Here's how the part is built. I have some questions about the finished solid (model axes, mm). Round coordinates to 2 decimals unless told otherwise and drop trailing zeros. Order: outer loops, then holes, each group sorted by start corner. A loop starts at its lowest first (then second) coordinate and runs counter-clockwise, first axis right, second up. Notation, with made-up numbers: (43.5, 79.5) -> (61.5, 79.5) arc R30 cw to (61.5, 118.5) -> close; hole circle Ø3 at (38, 79). An arc over 180 degrees is marked (long way). Answer in a Markdown table with one row per item.
```python
from build123d import *

# Parameters (mm, degrees)
SKETCH1_R               = 5.5499
EXTRUDE1_DEPTH          = 4.7625
SKETCH7_OUTSIDE_W       = 113.114
SKETCH7_OUTSIDE_H       = 115.816
SKETCH7_OUTSIDE_R       = 8.73125
EXTRUDE2_DEPTH          = 25.4
EXTRUDE2_DRAFT          = -60
MIRROR1_COPY_1_SKETCH_W = 113.114
MIRROR1_COPY_1_SKETCH_H = 115.816
MIRROR1_COPY_1_SKETCH_R = 8.73125
MIRROR1_COPY_1_DEPTH    = 25.4
MIRROR1_COPY_1_DRAFT    = -60


with BuildPart() as part:
    # Sketch1 → Extrude1 (new, symmetric)
    with BuildSketch(Plane.XY):
        Polygon((-8.73125, 5.040989538), (-8.73125, -5.040989538), (0, -10.081979076), (8.73125, -5.040989538), (8.73125, 5.040989538), (0, 10.081979076), align=None)
        with Locations(Location((0, 0, 0), (0, 0, 180))):
            Circle(SKETCH1_R, mode=Mode.SUBTRACT)
    extrude(amount=EXTRUDE1_DEPTH, both=True)


with BuildPart() as extrude2_tool:
    # Sketch7 outside → Extrude2 (with draft: the straight prism first)
    with BuildSketch(Plane.XY.offset(4.7625)):
        Rectangle(SKETCH7_OUTSIDE_W, SKETCH7_OUTSIDE_H)
        Circle(SKETCH7_OUTSIDE_R, mode=Mode.SUBTRACT)
    extrude(amount=-EXTRUDE2_DEPTH)
    # Extrude2: the draft: its side faces are tilted about the plane it starts from
    extrude2_sides = [extrude2_tool.faces().sort_by_distance(p)[0] for p in [
        (0, -57.908, -7.9375),
        (56.557, 0, -7.9375),
        (0, 57.908, -7.9375),
        (-56.557, 0, -7.9375),
        (-8.73125, 0, -7.9375),
    ]]
    draft(extrude2_sides, Plane.XY.offset(4.7625), EXTRUDE2_DRAFT)


with BuildPart() as part_1:
    add(part.part)

    # Extrude2: cut by extrude2_tool
    add(extrude2_tool.part, mode=Mode.SUBTRACT)


with BuildPart() as mirror1_copy_1_tool:
    # Mirror1 copy 1 sketch → Mirror1 copy 1 (with draft: the straight prism first)
    with BuildSketch(Plane(origin=(0, 0, -4.7625), x_dir=(1, 0, 0), z_dir=(0, 0, -1))):
        Rectangle(MIRROR1_COPY_1_SKETCH_W, MIRROR1_COPY_1_SKETCH_H)
        Circle(MIRROR1_COPY_1_SKETCH_R, mode=Mode.SUBTRACT)
    extrude(amount=-MIRROR1_COPY_1_DEPTH)
    # Mirror1 copy 1: the draft: its side faces are tilted about the plane it starts from
    mirror1_copy_1_sides = [mirror1_copy_1_tool.faces().sort_by_distance(p)[0] for p in [
        (0, -57.908, 7.9375),
        (56.557, 0, 7.9375),
        (0, 57.908, 7.9375),
        (-56.557, 0, 7.9375),
        (-8.73125, 0, 7.9375),
    ]]
    draft(mirror1_copy_1_sides, Plane(origin=(0, 0, -4.7625), x_dir=(1, 0, 0), z_dir=(0, 0, -1)), MIRROR1_COPY_1_DRAFT)


with BuildPart() as part_2:
    add(part_1.part)

    # Mirror1 copy 1: cut by mirror1_copy_1_tool
    add(mirror1_copy_1_tool.part, mode=Mode.SUBTRACT)


solid = part_2.part
```
1. Please list where these lines run through material, in increasing order: line 1 along X through (y, z) = (3.5, 1); line 2 along Y through (x, z) = (2.25, 2.75); line 3 along Y through (x, z) = (-4, 1).
Numbers:
| item | result |
|---|---|
| line 1 | x = -8.73 to -4.31, 4.31 to 8.73 |
| line 2 | y = -8.78 to -5.07, 5.07 to 8.78 |
| line 3 | y = -7.77 to -3.85, 3.85 to 7.77 |
2. Suppose I cut it at A-A on z = 3.5. Write out the boundary of the cut face in (x, y), then the cut area to 3 significant figures.
Numbers:
| item | result |
|---|---|
| outline | (-8.73, -5.04) -> (0, -10.08) -> (8.73, -5.04) -> (8.73, 5.04) -> (0, 10.08) -> (-8.73, 5.04) -> close; hole circle Ø11.1 at (0, 0) |
| area | 167 mm2 |
3. We'd pull the mould along Y, two halves only. Please class faces 1 (the face through (7.851, -4.507, -4.577)), 2 (the face through (0, -6, -4.762)), 3 (the face through (-2.561, 4.924, -0.067)), 4 (the face through (0.02, 9.05, 4.58)): released by +Y, released by -Y, zero draft, split by the parting line, or undercut.
Numbers:
| item | result |
|---|---|
| face 1 | released by -Y |
| face 2 | zero draft |
| face 3 | undercut |
| face 4 | released by +Y |
4. For pin 1 Ø6.5 at (x, y) = (0, 0) entering from -Z; pin 2 Ø5 at (x, z) = (-4, 0) entering from -Y, each with a flat end and sliding along its axis, tell me the tip position at first contact or that it passes through.
Numbers:
| item | result |
|---|---|
| pin 1 | passes through |
| pin 2 | stops at y = -9.22 |
